Read the model definition and answer for the solid it produces. Units are mm, in the model's axes. Coordinates: 2 decimals unless noted, no trailing zeros. Write each loop counter-clockwise with the first axis right and the second up, starting at its lowest first coordinate (ties: lowest second). Pieces come first, ordered by that corner, then holes. Notation, with made-up numbers: (14.5, 50) -> (48.5, 50) arc R17 ccw to (48.5, 54) -> close; hole circle Ø6 at (71.25, -40). An arc over 180 degrees is marked (long way). Answer as a JSON object with one key per item and string values. Group by question number.
(1) Find section B-B (x = -7.5). Give the vertices of the cut face in (y, z), then the cut area to 3 significant figures.
(2) Find section C-C (z = -16.45). Give the vertices of the cut face in (x, y), then the cut area to 3 significant figures.
(3) Find section A-A (y = 14.5). Give the vertices of the cut face in (x, z), then the cut area to 3 significant figures.
(4) Flat-ended cylindrical pins translate along their axes: P1, Ø1, axis at y = 10, z = -17.5, coming from the -X side; P2, Ø10, axis at x = 6, y = 15.5, coming from the -Z side. Find the tip coordinate at first contact, or state that the pin passes through.
(5) Straight lines are drawn through the part: L1, parallel to Z at x = 0, y = 5.5; L2, parallel to Z at x = -6.75, y = 16.25; L3, parallel to X at y = 13.25, z = -16.3. For each, find the intervals that lie inside material, in ascending order.
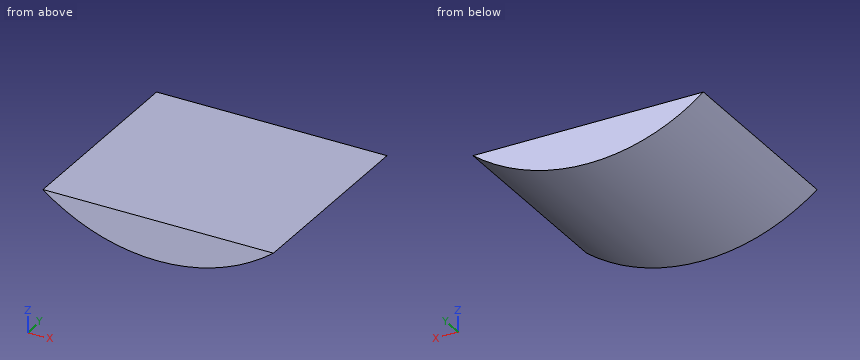
from build123d import *

# Parameters (mm, degrees)
SKETCH1_R               = 25.7
MAIN_CYLINDER_DEPTH     = 100
MAIN_START              = -98
MAIN_CUT_DOWN_DEPTH     = 98
BOSS_EXTRUDE1_DEPTH     = 20
CUT_EXTRUDE1_DEPTH      = 43.485056196
CUT_EXTRUDE1_DEPTH_BACK = 43.485056196
SKETCH9_W               = 59.759495022
SKETCH9_H               = 2


with BuildPart() as part:
    # Sketch1 → Main Cylinder (new body)
    with BuildSketch(Plane(origin=(0, 0, 0), x_dir=(1, 0, 0), z_dir=(0, 1, 0))):
        with Locations(Location((0, 0, 0), (0, 0, 270))):
            Circle(SKETCH1_R)
    extrude(amount=MAIN_CYLINDER_DEPTH)

    # Sketch4 → Main cut down (cut)
    with BuildSketch(Plane(origin=(0, 100, 0), x_dir=(1, 0, 0), z_dir=(0, 1, 0)).offset(MAIN_START)):
        with BuildLine():
            Line((-25.7, 0), (0, 0))
            Line((0, 0), (25.7, 0))
            ThreePointArc((25.7, 0), (0, 25.7), (-25.7, 0))
        make_face()
        with BuildLine():
            Line((25.7, 0), (0, 0))
            Line((0, 0), (-25.7, 0))
            ThreePointArc((-25.7, 0), (0, -25.7), (25.7, 0))
        make_face()
    extrude(amount=MAIN_CUT_DOWN_DEPTH, mode=Mode.SUBTRACT)

    # Sketch8 → Boss-Extrude1 (add)
    with BuildSketch(Plane(origin=(0, 2, 0), x_dir=(1, 0, 0), z_dir=(0, 1, 0))):
        with BuildLine():
            Line((-11.5075562, 14.8), (11.5075562, 14.8))
            ThreePointArc((11.5075562, 14.8), (0, 18.747369141), (-11.5075562, 14.8))
        make_face()
    extrude(amount=BOSS_EXTRUDE1_DEPTH)

    # Sketch9 → Cut-Extrude1 (cut, two sides: drawn at the far end of the back side and taken through both)
    with BuildSketch(Plane.XY.offset(-CUT_EXTRUDE1_DEPTH_BACK)):
        with Locations((-0.511377988, 1)):
            Rectangle(SKETCH9_W, SKETCH9_H)
    extrude(amount=CUT_EXTRUDE1_DEPTH + CUT_EXTRUDE1_DEPTH_BACK, mode=Mode.SUBTRACT)


solid = part.part
Results below:
{
 "1": {"outline": "(2, -17.18) -> (22, -17.18) -> (22, -14.8) -> (2, -14.8) -> close", "area": "47.6 mm2"},
 "2": {"outline": "(-8.99, 2) -> (8.99, 2) -> (8.99, 22) -> (-8.99, 22) -> close", "area": "360 mm2"},
 "3": {"outline": "(-11.51, -14.8) arc R18.75 ccw to (11.51, -14.8) -> close", "area": "62.0 mm2"},
 "4": {"P1": "stops at x = -7.9", "P2": "stops at z = -18.72"},
 "5": {"L1": "z = -18.75 to -14.8", "L2": "z = -17.49 to -14.8", "L3": "x = -9.26 to 9.26"}
}
